The model under review builds one solid part; all positions refer to its coordinate system, in mm. Face numbers are marked on the shaded views. Round coordinates to 2 decimals unless told otherwise and drop trailing zeros. Loops run counter-clockwise (first coordinate to the right, second up) from the corner with the lowest first, then second, coordinate; pieces in that order, holes last. Notation, with made-up numbers: M 28.25,47 L 32.25,47 A24 cw 32.25,63 Z; hole C 42.25,55.25 d6. An arc over 180 degrees is marked long. Return JSON: item names as keys, results as strings. Group by question number.
Q1. Consider section C-C (z = 6.75). Count the separate pieces of the cut face and the enclosed holes in it, and give its area (3 significant figures).
Q2. Consider section A-A (x = 49.44). State the section outline as (y, z) points.
Q3. Draft analysis for pull direction X (two halves, no side actions). For the marked faces 1 and 2, state which applies: pulls with the +X half, pulls with the -X half, needs draft (parallel to the pull), parting line crosses it, or undercut.
Q4. Clearance check with flat-ended pins moving along their axes: pin 1 Ø1.2 at (x, z) = (61, 5) entering from +Y; pin 2 Ø0.6 at (x, z) = (-34.5, 5) entering from +Y; pin 3 Ø0.6 at (y, z) = (-61.5, 3) entering from -X. State where each tip first meets the part, or that it passes through.
Q5. To check wall thickness, follow line 1 along Y through (x, z) = (-49.44, 6.75); line 2 along X through (y, z) = (0.5, 9.5); line 3 along Y through (x, z) = (-31.5, 8.5). State the ranges of each line that lie inside material, in increasing order.
from build123d import *

# Parameters (mm, degrees)
F0_R     = 8.25
F2_DEPTH = 10
F1_W     = 2
F1_H     = 2.2
F1_W_2   = 2.2
F3_DEPTH = 10


with BuildPart() as f2:
    # F0 (on Top) → F2 (new body)
    with BuildSketch(Plane.XY):
        with BuildLine():
            ThreePointArc((61.8, 59.8), (61.214214, 61.214214), (59.8, 61.8))
            Line((59.8, 61.8), (-59.8, 61.8))
            ThreePointArc((-59.8, 61.8), (-61.214214, 61.214214), (-61.8, 59.8))
            Line((-61.8, 59.8), (-61.8, -59.8))
            ThreePointArc((-61.8, -59.8), (-61.214214, -61.214214), (-59.8, -61.8))
            Line((-59.8, -61.8), (59.8, -61.8))
            ThreePointArc((59.8, -61.8), (61.214214, -61.214214), (61.8, -59.8))
            Line((61.8, -59.8), (61.8, 59.8))
        make_face()
        with Locations((-49.44, -49.44)):
            Circle(F0_R, mode=Mode.SUBTRACT)
        with Locations((-24.72, -49.44)):
            Circle(F0_R, mode=Mode.SUBTRACT)
        with Locations((-49.44, -24.72)):
            Circle(F0_R, mode=Mode.SUBTRACT)
        with Locations((-24.72, -24.72)):
            Circle(F0_R, mode=Mode.SUBTRACT)
        with Locations((0, -49.44)):
            Circle(F0_R, mode=Mode.SUBTRACT)
        with Locations((24.72, -49.44)):
            Circle(F0_R, mode=Mode.SUBTRACT)
        with Locations((49.44, -49.44)):
            Circle(F0_R, mode=Mode.SUBTRACT)
        with Locations((0, -24.72)):
            Circle(F0_R, mode=Mode.SUBTRACT)
        with Locations((24.72, -24.72)):
            Circle(F0_R, mode=Mode.SUBTRACT)
        with Locations((49.44, -24.72)):
            Circle(F0_R, mode=Mode.SUBTRACT)
        with Locations((-49.44, 0)):
            Circle(F0_R, mode=Mode.SUBTRACT)
        with Locations((-49.44, 24.72)):
            Circle(F0_R, mode=Mode.SUBTRACT)
        with Locations((-24.72, 0)):
            Circle(F0_R, mode=Mode.SUBTRACT)
        with Locations((-24.72, 24.72)):
            Circle(F0_R, mode=Mode.SUBTRACT)
        with Locations((-49.44, 49.44)):
            Circle(F0_R, mode=Mode.SUBTRACT)
        with Locations((-24.72, 49.44)):
            Circle(F0_R, mode=Mode.SUBTRACT)
        Circle(F0_R, mode=Mode.SUBTRACT)
        with Locations((24.72, 0)):
            Circle(F0_R, mode=Mode.SUBTRACT)
        with Locations((0, 24.72)):
            Circle(F0_R, mode=Mode.SUBTRACT)
        with Locations((24.72, 24.72)):
            Circle(F0_R, mode=Mode.SUBTRACT)
        with Locations((49.44, 0)):
            Circle(F0_R, mode=Mode.SUBTRACT)
        with Locations((49.44, 24.72)):
            Circle(F0_R, mode=Mode.SUBTRACT)
        with Locations((0, 49.44)):
            Circle(F0_R, mode=Mode.SUBTRACT)
        with Locations((24.72, 49.44)):
            Circle(F0_R, mode=Mode.SUBTRACT)
        with Locations((49.44, 49.44)):
            Circle(F0_R, mode=Mode.SUBTRACT)
    extrude(amount=F2_DEPTH)

    # F1 (on Top) → F3 (cut)
    with BuildSketch(Plane.XY):
        with Locations((-34.3, 61.8)):
            Rectangle(F1_W, F1_H)
        with Locations((34.3, 61.8)):
            Rectangle(F1_W_2, F1_H)
        with Locations((61.8, 34.3)):
            Rectangle(F1_W_2, F1_H)
        with Locations((61.8, -34.3)):
            Rectangle(F1_W_2, F1_H)
        with Locations((34.3, -61.8)):
            Rectangle(F1_W, F1_H)
        with Locations((-34.3, -61.8)):
            Rectangle(F1_W, F1_H)
        with Locations((-61.8, -34.3)):
            Rectangle(F1_W, F1_H)
        with Locations((-61.8, 34.3)):
            Rectangle(F1_W, F1_H)
    extrude(amount=F3_DEPTH, mode=Mode.SUBTRACT)


solid = f2.part
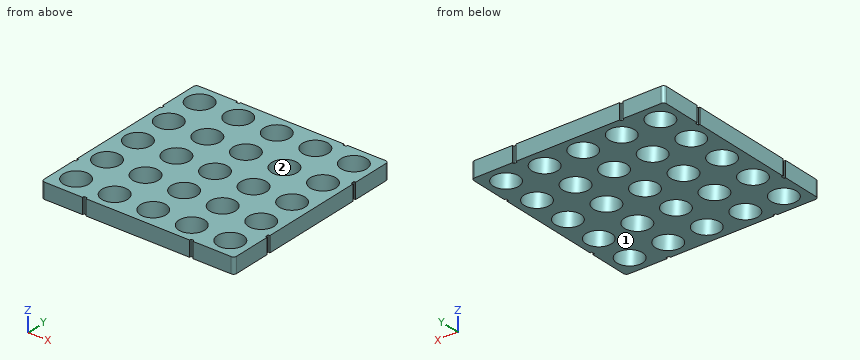
Values:
{
 "1": {"separate pieces": "1", "enclosed holes": "25", "area": "9,910 mm2"},
 "2": {"outline": "M -61.8,0 L -57.69,0 L -57.69,10 L -61.8,10 Z; M -41.19,0 L -32.97,0 L -32.97,10 L -41.19,10 Z; M -16.47,0 L -8.25,0 L -8.25,10 L -16.47,10 Z; M 8.25,0 L 16.47,0 L 16.47,10 L 8.25,10 Z; M 32.97,0 L 41.19,0 L 41.19,10 L 32.97,10 Z; M 57.69,0 L 61.8,0 L 61.8,10 L 57.69,10 Z"},
 "3": {"face 1": "needs draft", "face 2": "undercut"},
 "4": {"pin 1": "stops at y = 61.71", "pin 2": "stops at y = 60.7", "pin 3": "stops at x = -61.23"},
 "5": {"line 1": "y = -61.8 to -57.69, -41.19 to -32.97, -16.47 to -8.25, 8.25 to 16.47, 32.97 to 41.19, 57.69 to 61.8", "line 2": "x = -61.8 to -57.67, -41.21 to -32.95, -16.49 to -8.23, 8.23 to 16.49, 32.95 to 41.21, 57.67 to 61.8", "line 3": "y = -61.8 to -54.14, -44.74 to -29.42, -20.02 to -4.7, 4.7 to 20.02, 29.42 to 44.74, 54.14 to 61.8"}
}
